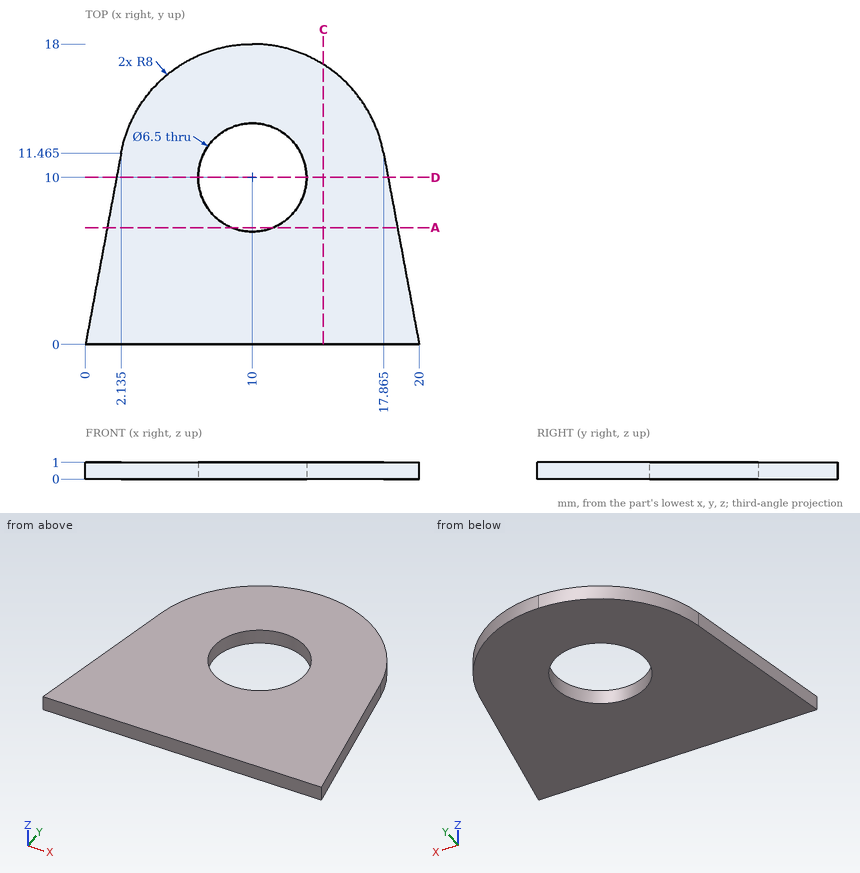
Here's the drawing with two shaded views (mm, measured from the low corner). I have some questions. Coordinates: 2 decimals unless noted, no trailing zeros. Write each loop counter-clockwise with the first axis right and the second up, starting at its lowest first coordinate (ties: lowest second). Pieces come first, ordered by that corner, then holes. Notation, with made-up numbers: M -38,52.25 L -10,52.25 A13 ccw -10,74.25 Z; hole C -37,-29 d10. An arc over 180 degrees is marked long. Use one line per item in the form item = value.
Q1. If we section it at C-C (x = 14.25): Write out the boundary of the cut face in (y, z), then the cut area to 3 significant figures.
Model answer:
outline = M 0,0 L 16.78,0 L 16.78,1 L 0,1 Z
area = 16.8 mm^2
Q2. If we section it at A-A (y = 7): Write out the boundary of the cut face in (x, z), then the cut area to 3 significant figures.
Model answer:
outline = M 1.3,0 L 8.75,0 L 8.75,1 L 1.3,1 Z; M 11.25,0 L 18.7,0 L 18.7,1 L 11.25,1 Z
area = 14.9 mm^2
Q3. If we section it at D-D (y = 10): Write out the boundary of the cut face in (x, z).
Model answer:
outline = M 1.86,0 L 6.75,0 L 6.75,1 L 1.86,1 Z; M 13.25,0 L 18.14,0 L 18.14,1 L 13.25,1 Z
Q4. I need wall thicknesses on line 1 along Y through (x, z) = (10, 0.75); line 2 along X through (y, z) = (10, 0.65); line 3 along Y through (x, z) = (11.5, 0.55). Which ranges of each line are inside material? Lowest first, please. Write a range as from..to.
Model answer:
line_1 = 0..6.75, 13.25..18
line_2 = 1.86..6.75, 13.25..18.14
line_3 = 0..7.12, 12.88..17.86
